Geometry check sheet. Reference: drawing and pictorial views, mm from the part's lowest x, y, z. A direction names the side the tool comes from. Round coordinates to 2 decimals unless told otherwise and drop trailing zeros. Loops run counter-clockwise (first coordinate to the right, second up) from the corner with the lowest first, then second, coordinate; pieces in that order, holes last. Notation, with made-up numbers: (55.25, 75) - (61.25, 75) arc R23 ccw to (61.25, 94) - close; hole circle Ø4 at (21.25, 75.5). An arc over 180 degrees is marked (long way). Answer in a Markdown table with one row per item. Add a question column.
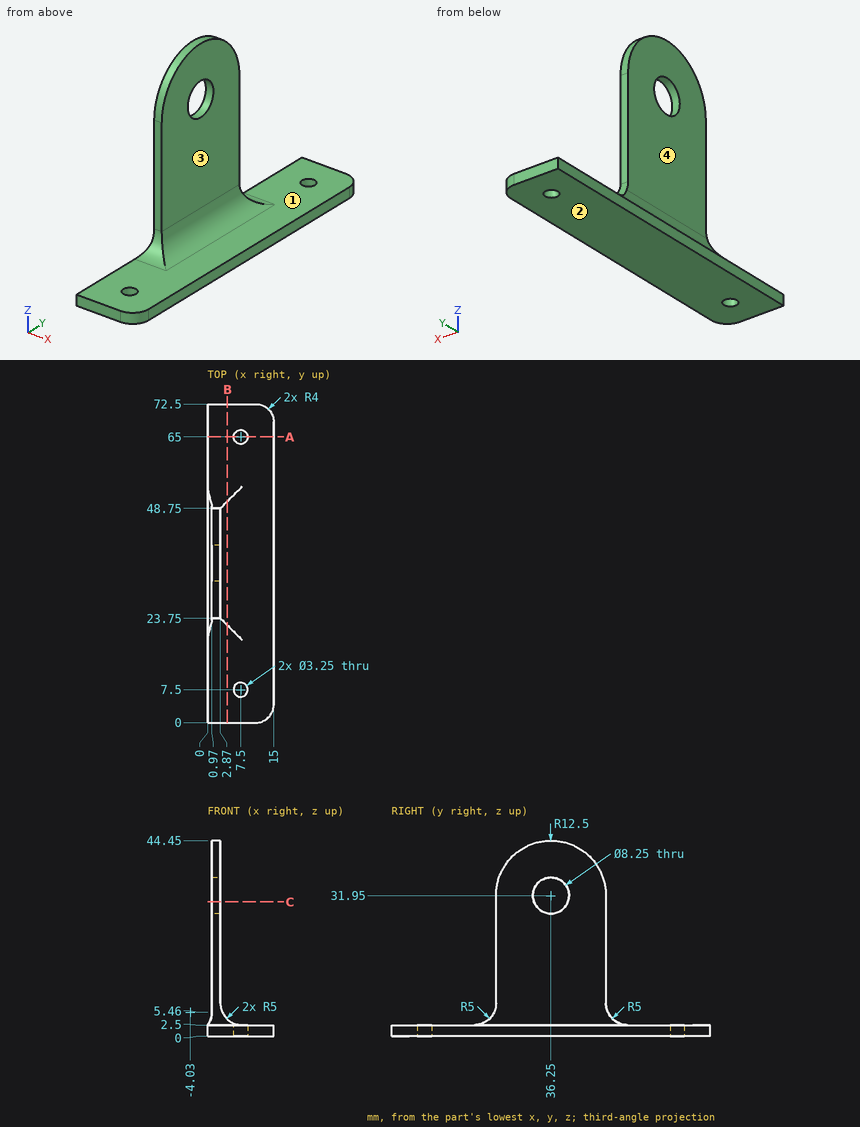
Q1. Depth check by flat-ended pin: P1, Ø0.6, axis at x = 2, z = 16, coming from the -Y side; P2, Ø0.6, axis at x = 1.5, z = 22.5, coming from the +Y side; P3, Ø13, axis at y = 36, z = 15.5, coming from the -X side. Enter the tip coordinate at first touch or a pass-through.
Q2. Cross-section at B-B, the plane x = 4.5. Enter the section's corners in (y, z).
Q3. Set-up check for the marked faces 1, 2, 3 and 4: record each of +Z, -Z, +X, -X, +Y, -Y from which the full face is reachable in a straight line by a thin tool's end or side.
Q4. Cross-section at C-C, the plane z = 30.5. Enter the section's corners in (x, y).
Q5. Cross-section at A-A, the plane y = 65. Enter the section's corners in (x, z) (1 decimal).
Q6. Scan lines: line 1 (Y direction, x = 7.5, z = 0.7) (1 decimal); line 2 (X direction, y = 65, z = 1.75) (1 decimal); line 3 (Z direction, x = 6, y = 63). Record each from-to range of solid material in increasing order. Write a range as from..to.
Check sheet entries:
| question | item | result |
|---|---|---|
| 1 | P1 | y = 23.75 |
| 1 | P2 | y = 48.75 |
| 1 | P3 | x = 0.97 |
| 2 | outline | (0, 0) - (72.5, 0) - (72.5, 2.5) - (53.75, 2.5) arc R5 cw to (50.38, 3.81) - (22.12, 3.81) arc R5 cw to (18.75, 2.5) - (0, 2.5) - close |
| 3 | face 1 | +Z, +X |
| 3 | face 2 | -Z, +X, -X, +Y, -Y |
| 3 | face 3 | +Z, +X, +Y, -Y |
| 3 | face 4 | +Z, -X, +Y, -Y |
| 4 | outline | (0.97, 23.75) - (2.87, 23.75) - (2.87, 32.39) - (0.97, 32.39) - close; (0.97, 40.11) - (2.87, 40.11) - (2.87, 48.75) - (0.97, 48.75) - close |
| 5 | outline | (0, 0) - (5.9, 0) - (5.9, 2.5) - (0, 2.5) - close; (9.1, 0) - (15, 0) - (15, 2.5) - (9.1, 2.5) - close |
| 6 | line 1 | 0..5.9, 9.1..63.4, 66.6..72.5 |
| 6 | line 2 | 0..5.9, 9.1..15 |
| 6 | line 3 | 0..2.5 |
